from build123d import *

# Parameters (mm, degrees)
EXTRUSION1_DEPTH                = 70
ESQUISSE2_W                     = 42
ESQUISSE2_H                     = 20
EXTRUSION2_DEPTH                = 70
ESQUISSE4_R                     = 1.5
EXTRUSION3_DEPTH                = 98.549987186
R_P_TITION_LIN_AIRE1_COUNT      = 2
R_P_TITION_LIN_AIRE1_PITCH      = 50
R_P_TITION_LIN_AIRE1_COUNT_DIR2 = 2
R_P_TITION_LIN_AIRE1_PITCH_DIR2 = 25
ESQUISSE5_R                     = 2
ENL_V_MAT_EXTRU_1_DEPTH         = 10
ESQUISSE6_R                     = 2
ENL_V_MAT_EXTRU_2_DEPTH         = 10
ESQUISSE7_R                     = 2
ENL_V_MAT_EXTRU_3_DEPTH         = 10
ESQUISSE8_R                     = 2
ENL_V_MAT_EXTRU_4_DEPTH         = 10


with BuildPart() as part:
    # Esquisse1 → Extrusion1 (new body)
    with BuildSketch(Plane.XY):
        Polygon((0, 0), (4, 0), (50, 0), (50, 4), (4, 4), (4, 50), (0, 50), align=None)
    extrude(amount=EXTRUSION1_DEPTH)

    # Esquisse2 → Extrusion2 (cut)
    with BuildSketch(Plane.ZY):
        with Locations((35, 40)):
            Rectangle(ESQUISSE2_W, ESQUISSE2_H)
    extrude(amount=-EXTRUSION2_DEPTH, mode=Mode.SUBTRACT)

    # Esquisse4 → Extrusion3 (cut, through all)
    with BuildSketch(Plane(origin=(0, 4, 0), x_dir=(1, 0, 0), z_dir=(0, 1, 0))):
        with Locations(Location((40, -60, 0), (0, 0, 270))):
            Circle(ESQUISSE4_R)
    extrusion3 = extrude(amount=-EXTRUSION3_DEPTH, mode=Mode.SUBTRACT)

    # Répétition linéaire1: Extrusion3 2 × 2
    with Locations(*[(-j * R_P_TITION_LIN_AIRE1_PITCH_DIR2, 0, -i * R_P_TITION_LIN_AIRE1_PITCH) for i in range(R_P_TITION_LIN_AIRE1_COUNT) for j in range(R_P_TITION_LIN_AIRE1_COUNT_DIR2) if (i, j) != (0, 0)]):
        add(extrusion3, mode=Mode.SUBTRACT)

    # Esquisse5 → Enlèv. mat.-Extru.1 (cut)
    with BuildSketch(Plane.ZY):
        with Locations((59.2, 45.5)):
            Circle(ESQUISSE5_R)
    extrude(amount=-ENL_V_MAT_EXTRU_1_DEPTH, mode=Mode.SUBTRACT)

    # Esquisse6 → Enlèv. mat.-Extru.2 (cut)
    with BuildSketch(Plane.ZY):
        with Locations((59.2, 34.5)):
            Circle(ESQUISSE6_R)
    extrude(amount=-ENL_V_MAT_EXTRU_2_DEPTH, mode=Mode.SUBTRACT)

    # Esquisse7 → Enlèv. mat.-Extru.3 (cut)
    with BuildSketch(Plane.ZY):
        with Locations((10.8, 34.5)):
            Circle(ESQUISSE7_R)
    extrude(amount=-ENL_V_MAT_EXTRU_3_DEPTH, mode=Mode.SUBTRACT)

    # Esquisse8 → Enlèv. mat.-Extru.4 (cut)
    with BuildSketch(Plane.ZY):
        with Locations((10.8, 45.5)):
            Circle(ESQUISSE8_R)
    extrude(amount=-ENL_V_MAT_EXTRU_4_DEPTH, mode=Mode.SUBTRACT)


solid = part.part
Check sheet for the modelled part. Datum: model origin and axes. Units: mm. A direction names the side the tool comes from. Coordinates: 2 decimals unless noted, no trailing zeros. Write each loop counter-clockwise with the first axis right and the second up, starting at its lowest first coordinate (ties: lowest second). Pieces come first, ordered by that corner, then holes. Notation, with made-up numbers: M 73,1 L 115,1 A24 cw 115,25 Z; hole C -23,42 d9. An arc over 180 degrees is marked long. Answer as CSV lines item,"result".
Q1. Go/stop test with flat-tipped pins: pin 1 (10 mm diameter, centred on y = 12.5, z = 17, fed in from -X); pin 2 (3.5 mm diameter, centred on y = 34.5, z = 59.2, fed in from -X); pin 3 (14 mm diameter, centred on y = 21, z = 24.5, fed in from +X); pin 4 (1 mm diameter, centred on x = 7, z = 52, fed in from +Y). Record where each tip stops, or that it passes through.
Check result:
pin 1,"x = 0"
pin 2,"through"
pin 3,"x = 4"
pin 4,"y = 4"
Q2. Set-up check for faces 1 (the face through (27, 4, 35)), 2 (the face through (2, 40, 14)), 3 (the face through (3, 14, 70)): record each of +Z, -Z, +X, -X, +Y, -Y from which the full face is reachable in a straight line by a thin tool's end or side.
Check result:
face 1,"+Z, -Z, +X, +Y"
face 2,"+X, -X, +Y"
face 3,"+Z, +X, -X, +Y, -Y"
Q3. Cross-section at C-C (z = 53). Record the boundary of the cut face in (x, y), then the cut area to 3 significant figures.
Check result:
outline,"M 0,0 L 50,0 L 50,4 L 4,4 L 4,30 L 0,30 Z"
area,"304 mm^2"
Q4. Cross-section at D-D (z = 60). Record the boundary of the cut face in (x, y), then the cut area to 3 significant figures.
Check result:
outline,"M 0,0 L 13.5,0 L 13.5,4 L 4,4 L 4,32.67 L 0,32.67 Z; M 0,36.33 L 4,36.33 L 4,43.67 L 0,43.67 Z; M 0,47.33 L 4,47.33 L 4,50 L 0,50 Z; M 16.5,0 L 38.5,0 L 38.5,4 L 16.5,4 Z; M 41.5,0 L 50,0 L 50,4 L 41.5,4 Z"
area,"331 mm^2"
Q5. Cross-section at B-B (y = 34.5). Record the boundary of the cut face in (x, z), then the cut area to 3 significant figures.
Check result:
outline,"M 0,0 L 4,0 L 4,8.8 L 0,8.8 Z; M 0,12.8 L 4,12.8 L 4,14 L 0,14 Z; M 0,56 L 4,56 L 4,57.2 L 0,57.2 Z; M 0,61.2 L 4,61.2 L 4,70 L 0,70 Z"
area,"80.0 mm^2"
Q6. Material ranges on probe 1 along X at (y, z) = (1.75, 10); probe 2 along Y at (x, z) = (2, 59); probe 3 along Y at (x, z) = (39.5, 12), recorded low to high. Write a range as from..to.
Check result:
probe 1,"0..13.5, 16.5..38.5, 41.5..50"
probe 2,"0..32.51, 36.49..43.51, 47.49..50"
probe 3,"0..4"
Q7. Mould release check, pull along Y, two halves, no side actions. Record for faces 4 (the face through (1.972, 32.726, 11.723)), 5 (the face through (1.972, 43.726, 11.723)), 6 (the face through (15.45, 2.03, 61.43)), 7 (the face through (2, 50, 63)): released by +Y, released by -Y, zero draft, split by the parting line, or undercut.
Check result:
face 4,"undercut"
face 5,"undercut"
face 6,"zero draft"
face 7,"released by +Y"
Q8. Cross-section at A-A (x = 40). Record the boundary of the cut face in (y, z).
Check result:
outline,"M 0,0 L 4,0 L 4,8.5 L 0,8.5 Z; M 0,11.5 L 4,11.5 L 4,58.5 L 0,58.5 Z; M 0,61.5 L 4,61.5 L 4,70 L 0,70 Z"
